Model file for the job. Use its own axes, mm. A direction names the side the tool comes from. Give positions to 0.01 mm unless a question says otherwise; leave off trailing zeros. Loops run counter-clockwise (first coordinate to the right, second up) from the corner with the lowest first, then second, coordinate; pieces in that order, holes last. Notation, with made-up numbers: M 72,6.5 L 124,6.5 A23 ccw 124,29.5 Z; hole C 36,39 d11. An arc over 180 degrees is marked long. Answer in a Markdown table with one row per item.
```python
from build123d import *

# Parameters (mm, degrees)
SKETCH1_W                                           = 3
SKETCH1_H                                           = 6.25
SKETCH2_R                                           = 1.5
SKETCH2_W                                           = 4
SKETCH2_H                                           = 4
CUT_EXTRUDE1_DEPTH                                  = 10
CSK_FOR_M3_COUNTERSUNK_FLAT_HEAD_SCREW1_D           = 3.4
CSK_FOR_M3_COUNTERSUNK_FLAT_HEAD_SCREW1_DEPTH       = 20.003
CSK_FOR_M3_COUNTERSUNK_FLAT_HEAD_SCREW1_CSINK_D     = 6.3
CSK_FOR_M3_COUNTERSUNK_FLAT_HEAD_SCREW1_CSINK_ANGLE = 90
CSK_FOR_M3_COUNTERSUNK_FLAT_HEAD_SCREW1_TIP         = 1.021463052


with BuildPart() as part:
    # Sketch1 → Base-Revolve (revolve)
    with BuildSketch(Plane.XY, mode=Mode.PRIVATE) as base_revolve_sk:
        with Locations((-1.5, 11.875)):
            Rectangle(SKETCH1_W, SKETCH1_H)
    revolve(base_revolve_sk.sketch.rotate(Axis((-34.925, 0, 0), (1, 0, 0)), 90), axis=Axis((-34.925, 0, 0), (1, 0, 0)))

    # Sketch2 → Cut-Extrude1 (cut)
    with BuildSketch(Plane(origin=(0, 0, 0), x_dir=(0, 0, -1), z_dir=(1, 0, 0))):
        with Locations((-11.875, 0)):
            Circle(SKETCH2_R)
        with Locations((11.875, 0)):
            Circle(SKETCH2_R)
        with Locations((0, 8.789946371)):
            Rectangle(SKETCH2_W, SKETCH2_H)
    extrude(amount=-CUT_EXTRUDE1_DEPTH, mode=Mode.SUBTRACT)

    # CSK for M3 Countersunk Flat Head Screw1
    with Locations(Plane(origin=(0, 0, 0), x_dir=(0, 0, -1), z_dir=(1, 0, 0))):
        with Locations((-11.875, 0), (11.875, 0)):
            CounterSinkHole(CSK_FOR_M3_COUNTERSUNK_FLAT_HEAD_SCREW1_D / 2, CSK_FOR_M3_COUNTERSUNK_FLAT_HEAD_SCREW1_CSINK_D / 2, depth=CSK_FOR_M3_COUNTERSUNK_FLAT_HEAD_SCREW1_DEPTH, counter_sink_angle=CSK_FOR_M3_COUNTERSUNK_FLAT_HEAD_SCREW1_CSINK_ANGLE)
            with Locations((0, 0, -(CSK_FOR_M3_COUNTERSUNK_FLAT_HEAD_SCREW1_DEPTH + CSK_FOR_M3_COUNTERSUNK_FLAT_HEAD_SCREW1_TIP / 2))):  # 118° drill point
                Cone(0, CSK_FOR_M3_COUNTERSUNK_FLAT_HEAD_SCREW1_D / 2, CSK_FOR_M3_COUNTERSUNK_FLAT_HEAD_SCREW1_TIP, mode=Mode.SUBTRACT)


solid = part.part
```
Q1. Saw through at C-C (y = -4). Give the cut face in (x, z), and give its area (3 significant figures).
Reported:
| item | result |
|---|---|
| outline | M -3,-14.46 L 0,-14.46 L 0,-7.78 L -3,-7.78 Z; M -3,7.78 L 0,7.78 L 0,14.46 L -3,14.46 Z |
| area | 40.0 mm² |
Q2. Drop flat-ended pins along their axis: pin 1 (10 mm diameter, centred on y = 8, z = 11, fed in from +X); pin 2 (3 mm diameter, centred on y = 0, z = -11.875, fed in from -X); pin 3 (1 mm diameter, centred on x = -0.5, y = 8, fed in from +Z); pin 4 (5.5 mm diameter, centred on y = 0, z = 11.875, fed in from +X). Give the stop position or say it passes through.
Reported:
| item | result |
|---|---|
| pin 1 | x = 0 |
| pin 2 | through |
| pin 3 | z = 12.99 |
| pin 4 | x = -0.4 |
Q3. Probe probe 1 along Y at (x, z) = (-0.95, 0); probe 2 along Z at (x, y) = (-0.9, 1); probe 3 along Y at (x, z) = (-2.35, -4). List the from-to ranges inside material, lowest first.
Reported:
| item | result |
|---|---|
| probe 1 | -15 to -8.75, 10.79 to 15 |
| probe 2 | -14.97 to -13.89, -9.86 to -8.69, 8.69 to 9.86, 13.89 to 14.97 |
| probe 3 | -14.46 to -7.78, 7.78 to 14.46 |
Q4. 3-axis set-ups, long thin cutter, end or side, ignore diameter. For faces 4 (the face through (-1, 10, 2)), 5 (the face through (-3, 6.5, -6.5)): which of +Z, -Z, +X, -X, +Y, -Y reach the whole face in a straight line?
Reported:
| item | result |
|---|---|
| face 4 | +X, -X |
| face 5 | +Z, -Z, -X, +Y, -Y |
Q5. Saw through at B-B (x = -2.45). Give the cut face in (y, z) (3 decimals), and give its area (3 significant figures).
Reported:
| item | result |
|---|---|
| outline | C 0,0 d30; hole C 0,-11.875 d3.4; hole C 0,11.875 d3.4; hole M 8.518,-2 L 10.79,-2 L 10.79,2 L 8.518,2 A8.75 ccw long Z |
| area | 440 mm² |
Q6. Mould opens along Z. For faces 1 (the face through (-1, 10.79, 0)), 2 (the face through (-1.48, -12.65, 8.06)), 3 (the face through (0, -9, 0)) say: released by +Z, released by -Z, zero draft, split by the parting line, or undercut.
Reported:
| item | result |
|---|---|
| face 1 | undercut |
| face 2 | split by the parting line |
| face 3 | zero draft |
Q7. Saw through at D-D (y = 1). Give the number of separate pieces and of enclosed holes in the cut face, and give its area (3 significant figures).
Reported:
| item | result |
|---|---|
| separate pieces | 4 |
| enclosed holes | 0 |
| area | 16.4 mm² |
Q8. Saw through at A-A (z = 0). Give the cut face in (x, y), and give its area (3 significant figures).
Reported:
| item | result |
|---|---|
| outline | M -3,-15 L 0,-15 L 0,-8.75 L -3,-8.75 Z; M -3,10.79 L 0,10.79 L 0,15 L -3,15 Z |
| area | 31.4 mm² |
